from build123d import *

# Parameters (mm, degrees)
F0_W     = 56.306915
F0_H     = 131.31
F1_DEPTH = 6.55
F2_R     = 5
F3_T     = -2.5


with BuildPart() as f1:
    # F0 (on Top) → F1 (new body)
    with BuildSketch(Plane.XY):
        with Locations((-6.374369, -1.911319)):
            Rectangle(F0_W, F0_H)
    extrude(amount=F1_DEPTH)

    # F2
    f2_edges = [f1.edges().sort_by_distance(p)[0] for p in [
        (21.779088, 63.743681, 3.275),
        (21.779088, -67.566319, 3.275),
        (-34.527827, -67.566319, 3.275),
        (-34.527827, 63.743681, 3.275),
    ]]
    fillet(f2_edges, radius=F2_R)

    # F3
    f3_openings = [f1.faces().sort_by_distance(p)[0] for p in [
        (-6.374369, -1.911319, 6.55),
    ]]
    offset(amount=F3_T, openings=f3_openings)


solid = f1.part
For this review, take the finished solid that the model builds, in its own axes (mm). A direction names the side the tool comes from. Coordinates: 2 decimals unless noted, no trailing zeros. Loops run counter-clockwise (first coordinate to the right, second up) from the corner with the lowest first, then second, coordinate; pieces in that order, holes last. Notation, with made-up numbers: (62.25, -15.75) - (109.25, -15.75) arc R19 cw to (109.25, 19.25) - close; hole circle Ø7 at (59, 51). An arc over 180 degrees is marked (long way). Use a Markdown table: item, result. Add a question column.
Item 1: We need section B-B (y = 52.5). Give the boundary of the cut face in (x, z), and give its area (3 significant figures).
Item 2: We need section C-C (x = -4.5). Give the boundary of the cut face in (y, z), and give its area (3 significant figures).
Item 3: Tool access review of faces 1 (the face through (-7, -65.066, 4)), 2 (the face through (-33.102, -66.063, 3.321)): name each direction out of +Z, -Z, +X, -X, +Y, -Y from which nothing blocks a thin tool from reaching the whole face with its end or side.
Item 4: We need section A-A (z = 4.5). Give the boundary of the cut face in (x, y).
Item 5: Mouldability with a two-part tool opening along X and no side actions: class faces 3 (the face through (-7, 63.744, 3)), 4 (the face through (20.353, 62.24, 3.321)), 5 (the face through (-31.315, 60.492, 4.553)) as pulls with the +X half, pulls with the -X half, needs draft (parallel to the pull), parting line crosses it, or undercut.
Item 6: Insertion check: pin 1 Ø2 at (x, y) = (-3, 45) entering from +Z. The pin has a flat end and moves straight along its axis. Give the tip position at first contact, or say it passes through.
Item 7: For line 1 (Y direction, x = 4, z = 3.75); line 2 (X direction, y = -61, z = 5.25); line 3 (Z direction, x = -19, y = -18), list the stretches that pass through material, from the lowest coordinate up.
Results list:
| question | item | result |
|---|---|---|
| 1 | outline | (-34.53, 0) - (21.78, 0) - (21.78, 6.55) - (19.28, 6.55) - (19.28, 2.5) - (-32.03, 2.5) - (-32.03, 6.55) - (-34.53, 6.55) - close |
| 1 | area | 161 mm^2 |
| 2 | outline | (-67.57, 0) - (63.74, 0) - (63.74, 6.55) - (61.24, 6.55) - (61.24, 2.5) - (-65.07, 2.5) - (-65.07, 6.55) - (-67.57, 6.55) - close |
| 2 | area | 349 mm^2 |
| 3 | face 1 | +Z |
| 3 | face 2 | +Z, -Z, -X, -Y |
| 4 | outline | (-34.53, -62.57) arc R5 ccw to (-29.53, -67.57) - (16.78, -67.57) arc R5 ccw to (21.78, -62.57) - (21.78, 58.74) arc R5 ccw to (16.78, 63.74) - (-29.53, 63.74) arc R5 ccw to (-34.53, 58.74) - close; hole (-32.03, -62.57) arc R2.5 ccw to (-29.53, -65.07) - (16.78, -65.07) arc R2.5 ccw to (19.28, -62.57) - (19.28, 58.74) arc R2.5 ccw to (16.78, 61.24) - (-29.53, 61.24) arc R2.5 ccw to (-32.03, 58.74) - close |
| 5 | face 3 | needs draft |
| 5 | face 4 | pulls with the +X half |
| 5 | face 5 | undercut |
| 6 | pin 1 | stops at z = 2.5 |
| 7 | line 1 | y = -67.57 to -65.07, 61.24 to 63.74 |
| 7 | line 2 | x = -34.53 to -32.03, 19.28 to 21.78 |
| 7 | line 3 | z = 0 to 2.5 |
